Verification items for this drawing (mm, ordinates from the low corner). A direction names the side the tool comes from. Round coordinates to 2 decimals unless told otherwise and drop trailing zeros. Write each loop counter-clockwise with the first axis right and the second up, starting at its lowest first coordinate (ties: lowest second). Pieces come first, ordered by that corner, then holes. Notation, with made-up numbers: (-9, -37) -> (33, -37) arc R36 cw to (33, 2) -> close; hole circle Ø7 at (82.25, 67.25). An arc over 180 degrees is marked (long way). Return JSON: item names as keys, results as strings. Group by question number.
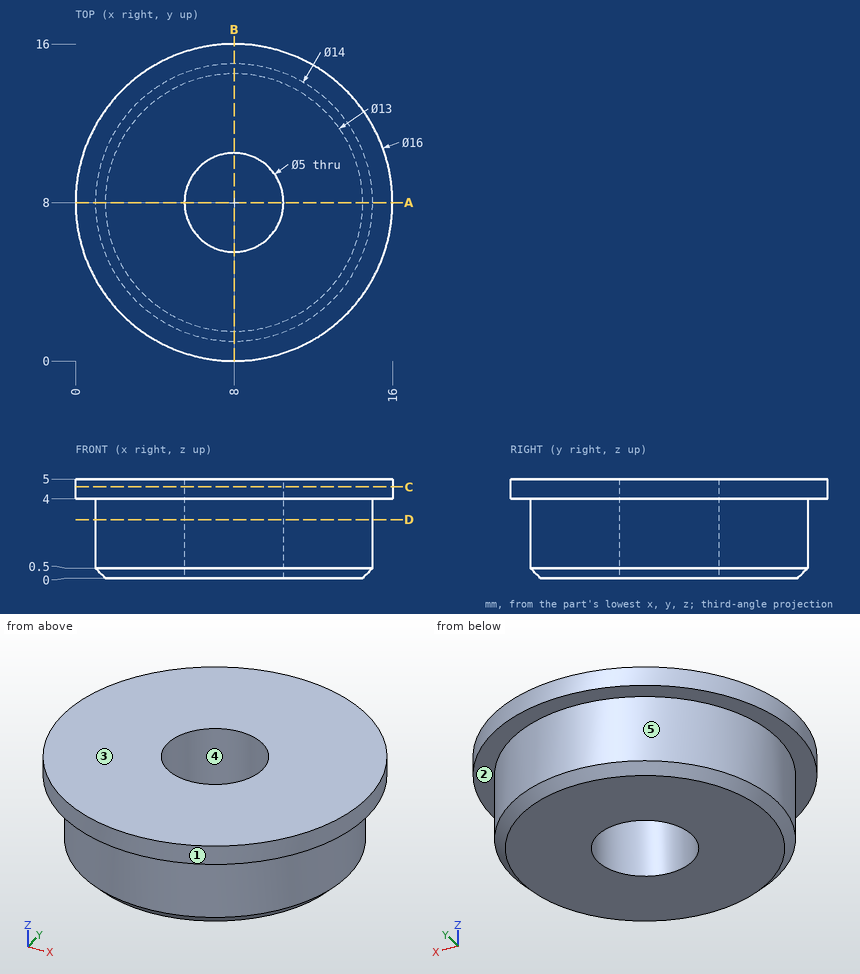
1) Sectioned sample at D-D on z = 2.95. Enter the section's corners in (x, y), and give its area (3 significant figures).
2) Material ranges on probe 1 along Y at (x, z) = (8, 2.25); probe 2 along Z at (x, y) = (15.25, 7.75); probe 3 along Y at (x, z) = (8.75, 3.75), recorded low to high. Write a range as [from, to].
3) Go/stop test with flat-tipped pins: P1, Ø1.5, axis at x = 4.5, z = 2.5, coming from the -Y side; P2, Ø3, axis at y = 8.5, z = 1.5, coming from the -X side. Record where each tip stops, or that it passes through.
4) Tool access check on the marked faces 1 and 2. Record the directions out of +Z, -Z, +X, -X, +Y, -Y that give a thin tool (end or side, any length) a straight path to the whole face; none if there is none.
5) Sectioned sample at C-C on z = 4.6. Enter the section's corners in (x, y), and give its area (3 significant figures).
6) Mould release check, pull along Y, two halves, no side actions. Record for the marked faces 3, 4 and 5: +Y half, -Y half, draft (parallel to the pull), parting line (faces both ways), or undercut.
7) Sectioned sample at A-A on y = 8. Enter the section's corners in (x, z).
Evaluation:
{
 "1": {"outline": "circle Ø14 at (8, 8); hole circle Ø5 at (8, 8)", "area": "134 mm2"},
 "2": {"probe 1": "y = [1, 5.5], [10.5, 15]", "probe 2": "z = [4, 5]", "probe 3": "y = [1.04, 5.62], [10.38, 14.96]"},
 "3": {"P1": "stops at y = 1.56", "P2": "stops at x = 1"},
 "4": {"face 1": "+Z, -Z", "face 2": "-Z"},
 "5": {"outline": "circle Ø16 at (8, 8); hole circle Ø5 at (8, 8)", "area": "181 mm2"},
 "6": {"face 3": "draft", "face 4": "undercut", "face 5": "parting line"},
 "7": {"outline": "(0, 4) -> (1, 4) -> (1, 0.5) -> (1.5, 0) -> (5.5, 0) -> (5.5, 5) -> (0, 5) -> close; (10.5, 0) -> (14.5, 0) -> (15, 0.5) -> (15, 4) -> (16, 4) -> (16, 5) -> (10.5, 5) -> close"}
}
